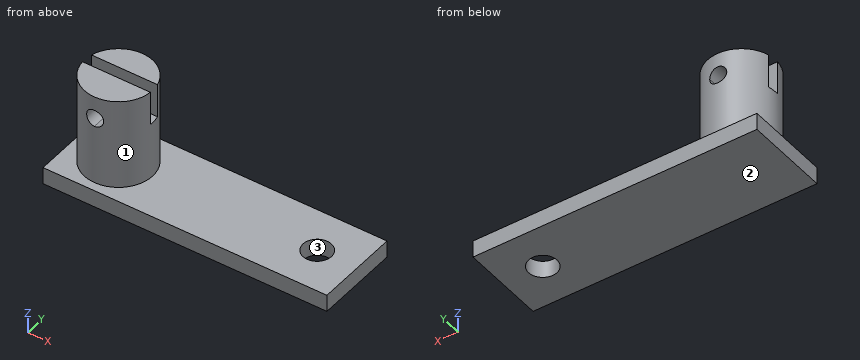
```python
from build123d import *

# Parameters (mm, degrees)
F0_W     = 50
F0_H     = 15
F0_R     = 6
F0_R_2   = 2.5
F1_DEPTH = 3
F2_R     = 6
F3_DEPTH = 19
F6_DEPTH = 6
F9_DEPTH = 25


with BuildPart() as f1:
    # F0 (on Top) → F1 (new body)
    with BuildSketch(Plane.XY):
        with Locations((25, 7.5)):
            Rectangle(F0_W, F0_H)
        with Locations((8, 7.5)):
            Circle(F0_R, mode=Mode.SUBTRACT)
        with Locations((43, 7.5)):
            Circle(F0_R_2, mode=Mode.SUBTRACT)
        with Locations((8, 7.5)):
            Circle(F0_R)
    extrude(amount=F1_DEPTH)

    # F2 (on Top) → F3 (join)
    with BuildSketch(Plane.XY):
        with Locations((8, 7.5)):
            Circle(F2_R)
    extrude(amount=F3_DEPTH)

    # F5 (on offset) → F6 (cut)
    with BuildSketch(Plane.XY.offset(19)):
        Polygon((0, 8), (0, 7), (14.8029690608, 7), (14.8029690608, 8.9999996126), (0, 8.9999996126), align=None)
    extrude(amount=-F6_DEPTH, mode=Mode.SUBTRACT)

    # F8 (on offset) → F9 (cut)
    with BuildSketch(Plane.XZ):
        with BuildLine():
            ThreePointArc((8, 13.5), (9.0606601718, 13.9393398282), (9.5, 15))
            ThreePointArc((9.5, 15), (6.9393398282, 16.0606601718), (8, 13.5))
        make_face()
    extrude(amount=-F9_DEPTH, mode=Mode.SUBTRACT)


solid = f1.part
```
Work out the finished part from the listing and answer in its coordinate system (mm). Face numbers are marked on the shaded views. Give positions to 0.01 mm unless a question says otherwise; leave off trailing zeros. Write each loop counter-clockwise with the first axis right and the second up, starting at its lowest first coordinate (ties: lowest second). Pieces come first, ordered by that corner, then holes. Notation, with made-up numbers: (27, 68) -> (65, 68) arc R13 ccw to (65, 75) -> close; hole circle Ø7 at (41, 12.5). An arc over 180 degrees is marked (long way). Write each question's results on one line, items separated by ' | '.
1. Determine the mould class of the marked faces 1, 2 and 3 for opening direction X: +X half, -X half, draft (parallel to the pull), parting line (faces both ways), or undercut.
Data:
face 1: parting line | face 2: draft | face 3: undercut
2. Find section C-C on y = 11.5. Determine the outline of the cut face in (x, z).
Data:
outline: (0, 0) -> (50, 0) -> (50, 3) -> (12.47, 3) -> (12.47, 19) -> (3.53, 19) -> (3.53, 3) -> (0, 3) -> close; hole circle Ø3 at (8, 15)
3. Find section B-B on x = 43. Determine the outline of the cut face in (y, z), and give its area (3 significant figures).
Data:
outline: (0, 0) -> (5, 0) -> (5, 3) -> (0, 3) -> close; (10, 0) -> (15, 0) -> (15, 3) -> (10, 3) -> close | area: 30.0 mm^2
4. Each of these flat-tipped pins is pushed along its axis until it touches: pin 1 Ø7.5 at (x, y) = (20.5, 7.5) entering from +Z; pin 2 Ø3.5 at (x, z) = (8, 15) entering from +Y; pin 3 Ø4 at (y, z) = (7.5, 9.5) entering from -X; pin 4 Ø4.5 at (x, y) = (43, 7.5) entering from -Z. Where does it stop, or does it pass through?
Data:
pin 1: z = 3 | pin 2: y = 13.5 | pin 3: x = 2 | pin 4: through
5. Find section D-D on x = 37. Determine the outline of the cut face in (y, z), and give its area (3 significant figures).
Data:
outline: (0, 0) -> (15, 0) -> (15, 3) -> (0, 3) -> close | area: 45.0 mm^2
6. Straight lines are drawn through the part: L1, parallel to Z at x = 8, y = 5.4; L2, parallel to Y at x = 43, z = 1.35; L3, parallel to Z at x = 43, y = 1. For each, find the intervals that lie inside material, in ascending order.
Data:
L1: 0 to 13.5, 16.5 to 19 | L2: 0 to 5, 10 to 15 | L3: 0 to 3
7. Find section A-A on y = 7.5. Determine the outline of the cut face in (x, z), and give its area (3 significant figures).
Data:
outline: (0, 0) -> (40.5, 0) -> (40.5, 3) -> (14, 3) -> (14, 13) -> (2, 13) -> (2, 3) -> (0, 3) -> close; (45.5, 0) -> (50, 0) -> (50, 3) -> (45.5, 3) -> close | area: 255 mm^2
